Answer from the drawing. Dimensions are ordinates in mm from the lowest x, y and z of the part. A direction names the side the tool comes from. Give positions to 0.01 mm unless a question says otherwise; leave off trailing zeros. Order: outer loops, then holes, each group sorted by start corner. A loop starts at its lowest first (then second) coordinate and runs counter-clockwise, first axis right, second up. Notation, with made-up numbers: (52.5, 89.5) - (89.5, 89.5) arc R9 cw to (89.5, 106.5) - close; hole circle Ø3 at (-20.5, -24). An arc over 180 degrees is marked (long way). Write each question's results on one line, items separated by ' | '.
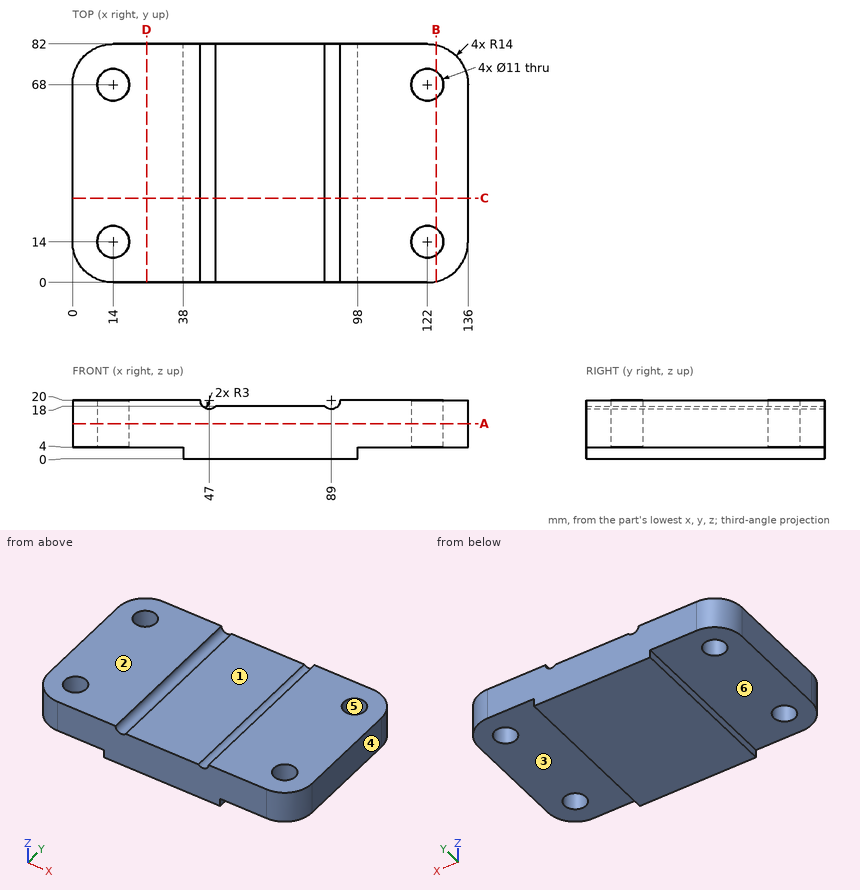
1. Straight lines are drawn through the part: line 1 (Y direction, x = 14, z = 15.75); line 2 (X direction, y = 68, z = 9); line 3 (X direction, y = 72.5, z = 14.5). For each, find the intervals that lie inside material, in ascending order. Write a range as [from, to].
Answer list:
line 1: [0, 8.5], [19.5, 62.5], [73.5, 82] | line 2: [0, 8.5], [19.5, 116.5], [127.5, 136] | line 3: [0.74, 10.84], [17.16, 118.84], [125.16, 135.26]
2. A cutting plane is placed at B-B, the plane x = 125. Write down the section's boundary in (y, z).
Answer list:
outline: (0.33, 4) - (9.39, 4) - (9.39, 20) - (0.33, 20) - close; (18.61, 4) - (63.39, 4) - (63.39, 20) - (18.61, 20) - close; (72.61, 4) - (81.67, 4) - (81.67, 20) - (72.61, 20) - close
3. A tool of negligible diameter and unlimited length cuts with its end or side. For the marked faces 1, 2 and 3, from which of +Z, -Z, +X, -X, +Y, -Y can it reach the whole face along a straight path? Write none if from no direction.
Answer list:
face 1: +Z, +Y, -Y | face 2: +Z, +X, -X, +Y, -Y | face 3: -Z, +X, +Y, -Y
4. A cutting plane is placed at D-D, the plane x = 25.5. Write down the section's boundary in (y, z), then the cut area to 3 significant figures.
Answer list:
outline: (0, 4) - (82, 4) - (82, 20) - (0, 20) - close | area: 1,310 mm^2
5. Determine the mould class of the marked faces 4, 5 and 6 for opening direction X: +X half, -X half, draft (parallel to the pull), parting line (faces both ways), or undercut.
Answer list:
face 4: +X half | face 5: undercut | face 6: draft
6. A cutting plane is placed at C-C, the plane y = 29. Write down the section's boundary in (x, z).
Answer list:
outline: (0, 4) - (38, 4) - (38, 0) - (98, 0) - (98, 4) - (136, 4) - (136, 20) - (92, 20) arc R3 cw to (86.76, 18) - (49.24, 18) arc R3 cw to (44, 20) - (0, 20) - close
7. A cutting plane is placed at A-A, the plane z = 12. Write down the section's boundary in (x, y).
Answer list:
outline: (0, 14) arc R14 ccw to (14, 0) - (122, 0) arc R14 ccw to (136, 14) - (136, 68) arc R14 ccw to (122, 82) - (14, 82) arc R14 ccw to (0, 68) - close; hole circle Ø11 at (14, 14); hole circle Ø11 at (14, 68); hole circle Ø11 at (122, 14); hole circle Ø11 at (122, 68)
8. Given P1, Ø1, axis at x = 28, y = 26.5, coming from the -Z side; P2, Ø3, axis at y = 23.5, z = 1, coming from the +X side; P3, Ø19, axis at x = 66, y = 29.5, coming from the +Z side, each flat-ended and moving along its own axis, determine where each tip first touches the part or whether it passes through.
Answer list:
P1: z = 4 | P2: x = 98 | P3: z = 18
